For this review, use the dimensioned drawing (mm, ordinates from the lowest corner) and the shaded views. A direction names the side the tool comes from. Give positions to 0.01 mm unless a question says otherwise; leave off trailing zeros. Write each loop counter-clockwise with the first axis right and the second up, starting at its lowest first coordinate (ties: lowest second). Pieces come first, ordered by that corner, then holes.
1) For P1, Ø1, axis at x = 82, y = 49.5, coming from the -Z side; P2, Ø2, axis at x = 52, z = 40.5, coming from the +Y side; P3, Ø10, axis at x = 19, z = 52, coming from the +Y side, all flat-tipped, find the tip position at first contact; note any pin that passes through.
2) We need section D-D on x = 30.5. Give the boundary of the cut face in (y, z).
3) Machinability: for the marked faces 1 and 2, which of the approach directions +Z, -Z, +X, -X, +Y, -Y give a long, thin tool a straight path to every point of the face, cutting with its end or side? Answer none if there is none.
4) We need section C-C on z = 54. Give the boundary of the cut face in (x, y).
5) We need section A-A on x = 89. Give the boundary of the cut face in (y, z), and give its area (3 significant figures).
6) We need section B-B on y = 46.5. Give the boundary of the cut face in (x, z).
7) Wall thickness on line 1 along Y through (x, z) = (62, 33.5); line 2 along Z through (x, y) = (38, 25.5); line 3 along Y through (x, z) = (96.5, 17.5): over which ranges is each line inside the solid? List them lowest first.
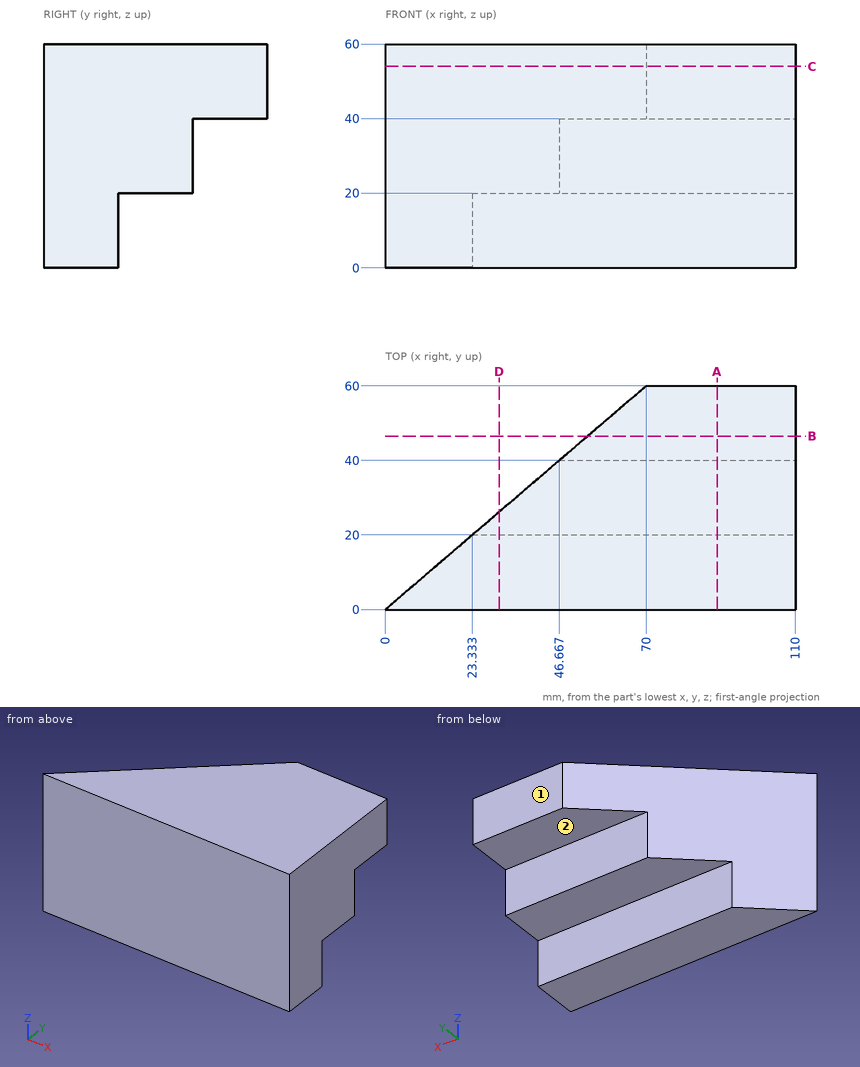
Results list:
1. P1: stops at z = 40
1. P2: stops at y = 45.43
1. P3: stops at y = 20.57
2. outline: (0, 0) - (20, 0) - (20, 20) - (26.14, 20) - (26.14, 60) - (0, 60) - close
3. face 1: +Z, -Z, +X, -X, +Y
3. face 2: -Z, +X, -X, +Y
4. outline: (0, 0) - (110, 0) - (110, 60) - (70, 60) - close
5. outline: (0, 0) - (20, 0) - (20, 20) - (40, 20) - (40, 40) - (60, 40) - (60, 60) - (0, 60) - close
5. area: 2,400 mm2
6. outline: (54.25, 40) - (110, 40) - (110, 60) - (54.25, 60) - close
7. line 1: y = 0 to 40
7. line 2: z = 20 to 60
7. line 3: y = 0 to 20
